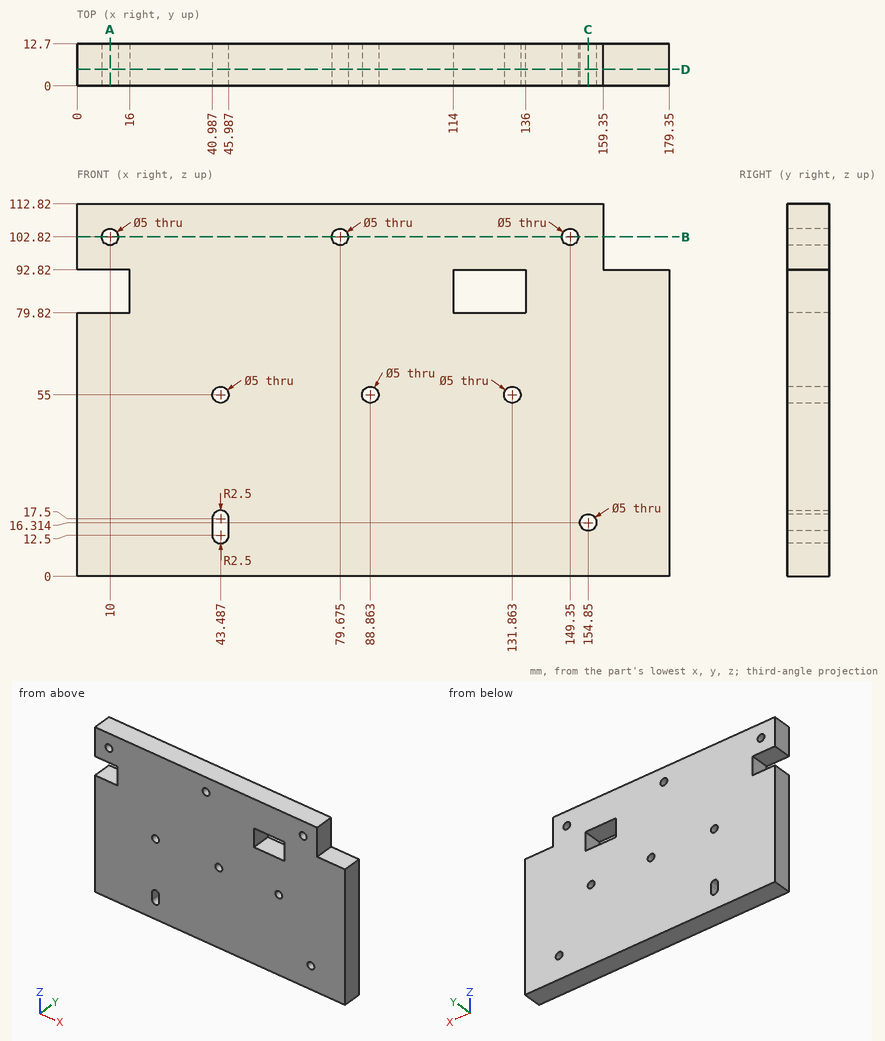
Geometry check sheet. Reference: drawing and pictorial views, mm from the part's lowest x, y, z. Give positions to 0.01 mm unless a question says otherwise; leave off trailing zeros. Order: outer loops, then holes, each group sorted by start corner. A loop starts at its lowest first (then second) coordinate and runs counter-clockwise, first axis right, second up. Notation, with made-up numbers: M 17.25,-8.75 L 37.25,-8.75 A19 ccw 37.25,8.25 Z; hole C 53,43 d8. An arc over 180 degrees is marked long. Use one line per item in the form item = value. Start each with the question number.
Q1. Section check C-C (x = 154.85). Enter the section's corners in (y, z), then the cut area to 3 significant figures.
Q2. Scan lines: line 1 along X through (y, z) = (5.75, 102.82) (3 decimals); line 2 along Z through (x, y) = (119, 3.25); line 3 along X through (y, z) = (6, 55). Record each from-to range of solid material in increasing order. Write a range as [from, to].
Q3. Section check D-D (y = 5). Count the separate pieces of the cut face and the enclosed holes in it, then the cut area to 3 significant figures.
Q4. Section check B-B (z = 102.82). Enter the section's corners in (x, y) (3 decimals).
Q5. Go/stop test with flat-tipped pins: pin 1 Ø5 at (x, y) = (63.5, 8) entering from -Z; pin 2 Ø4.5 at (x, z) = (149.35, 102.82) entering from -Y; pin 3 Ø6.5 at (y, z) = (6, 105) entering from +X; pin 4 Ø6.5 at (x, y) = (166, 8.5) entering from +Z. Record where each tip stops, or that it passes through.
Q6. Section check A-A (x = 10). Enter the section's corners in (y, z).
Evaluation:
q1.outline = M 0,0 L 12.7,0 L 12.7,13.81 L 0,13.81 Z; M 0,18.81 L 12.7,18.81 L 12.7,112.82 L 0,112.82 Z
q1.area = 1,370 mm2
q2.line_1 = [0, 7.5], [12.5, 77.175], [82.175, 146.85], [151.85, 159.35]
q2.line_2 = [0, 79.82], [92.82, 112.82]
q2.line_3 = [0, 40.99], [45.99, 86.36], [91.36, 129.36], [134.36, 179.35]
q3.separate_pieces = 1
q3.enclosed_holes = 9
q3.area = 19,200 mm2
q4.outline = M 0,0 L 7.5,0 L 7.5,12.7 L 0,12.7 Z; M 12.5,0 L 77.175,0 L 77.175,12.7 L 12.5,12.7 Z; M 82.175,0 L 146.85,0 L 146.85,12.7 L 82.175,12.7 Z; M 151.85,0 L 159.35,0 L 159.35,12.7 L 151.85,12.7 Z
q5.pin_1 = 0
q5.pin_2 = through
q5.pin_3 = 159.35
q5.pin_4 = 92.82
q6.outline = M 0,0 L 12.7,0 L 12.7,79.82 L 0,79.82 Z; M 0,92.82 L 12.7,92.82 L 12.7,100.32 L 0,100.32 Z; M 0,105.32 L 12.7,105.32 L 12.7,112.82 L 0,112.82 Z
